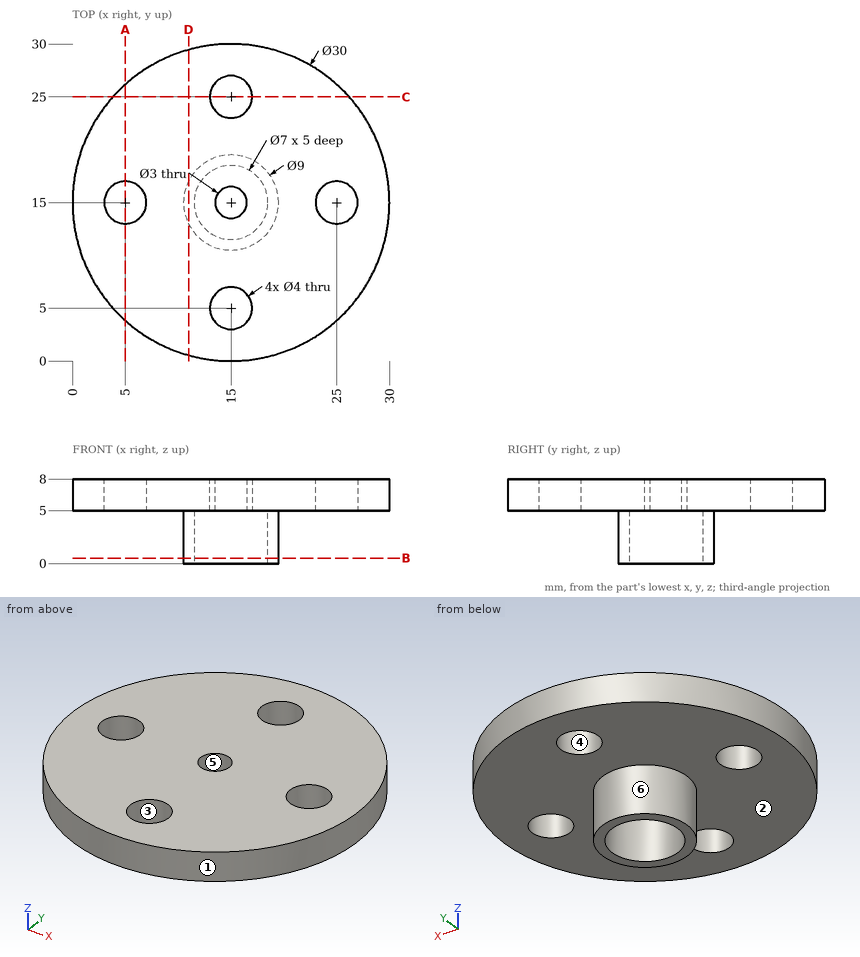
Check sheet for the drawn part. Datum: minimum x, y, z corner. Units: mm. A direction names the side the tool comes from. Round coordinates to 2 decimals unless told otherwise and drop trailing zeros. Write each loop counter-clockwise with the first axis right and the second up, starting at its lowest first coordinate (ties: lowest second). Pieces come first, ordered by that corner, then holes. Notation, with made-up numbers: (-8, 49.25) -> (30, 49.25) arc R19 ccw to (30, 62.25) -> close; hole circle Ø9 at (55, 82). An arc over 180 degrees is marked (long way). Write each question's results on one line, items separated by ' | '. Start each with the question number.
1. Cross-section at D-D (x = 11). Enter the section's corners in (y, z), then the cut area to 3 significant figures.
2. Cross-section at A-A (x = 5). Enter the section's corners in (y, z).
3. Material ranges on probe 1 along Y at (x, z) = (15, 6.9); probe 2 along Y at (x, z) = (15, 1.55); probe 3 along X at (y, z) = (14, 5.75), recorded low to high. Write a range as from..to.
4. Draft check along X on the marked faces 1, 2, 3 and 4. Enter one of: +X half, -X half, draft (parallel to the pull), parting line (faces both ways), or undercut.
5. Set-up check for the marked faces 5 and 6: record each of +Z, -Z, +X, -X, +Y, -Y from which the full face is reachable in a straight line by a thin tool's end or side.
6. Cross-section at B-B (z = 0.5). Enter the section's corners in (x, y), then the cut area to 3 significant figures.
7. Depth check by flat-ended pin: P1, Ø3.5, axis at x = 15, y = 5, coming from the +Z side; P2, Ø3.5, axis at x = 15, y = 15, coming from the -Z side; P3, Ø1.5, axis at y = 11.5, z = 2, coming from the -X side. Enter the tip coordinate at first touch or a pass-through.
Solutions:
1) outline: (0.54, 5) -> (12.94, 5) -> (12.94, 0) -> (17.06, 0) -> (17.06, 5) -> (29.46, 5) -> (29.46, 8) -> (0.54, 8) -> close | area: 107 mm2
2) outline: (3.82, 5) -> (13, 5) -> (13, 8) -> (3.82, 8) -> close; (17, 5) -> (26.18, 5) -> (26.18, 8) -> (17, 8) -> close
3) probe 1: y = 0..3, 7..13.5, 16.5..23, 27..30 | probe 2: y = 10.5..11.5, 18.5..19.5 | probe 3: x = 0.03..3.27, 6.73..13.88, 16.12..23.27, 26.73..29.97
4) face 1: parting line | face 2: draft | face 3: undercut | face 4: undercut
5) face 5: +Z, -Z | face 6: -Z
6) outline: circle Ø9 at (15, 15); hole circle Ø7 at (15, 15) | area: 25.1 mm2
7) P1: passes through | P2: stops at z = 5 | P3: stops at x = 11.44
